Autodesk Inventor part; units mm, degrees
ref_plane "YZ Plane" through (0, 0, 0) normal (1, 0, 0) x (0, 1, 0)
ref_plane "XZ Plane" through (0, 0, 0) normal (0, 1, 0) x (-1, 0, 0)
ref_plane "XY Plane" through (0, 0, 0) normal (0, 0, 1) x (1, 0, 0)
sketch "Sketch1" plane through (0, 0, 0) normal (0, 1, 0) x (-1, 0, 0)
  line L0 (-81, 62) -> (81, 62)
  line L1 (81, 62) -> (81, -62)
  line L2 (81, -62) -> (-81, -62)
  line L3 (-81, -62) -> (-81, 62)
  point P0 (0, 0)
  dimension "d117" = 124
  dimension "d118" = 162
  dimension "d119" = 81
  dimension "d120" = 62
extrude "Extrusion1" add sketch "Sketch1" along normal blind 5
fillet "Fillet1" radius 5 4 edges at (81, 2.5, 62) (81, 2.5, -62) (-81, 2.5, -62) (-81, 2.5, 62)
sketch "Sketch3" plane through (0, 5, 0) normal (0, 1, 0) x (1, 0, 0)
  circle A0 centre (74, -55) radius 3
  circle A1 centre (-74, -55) radius 3
  circle A2 centre (-74, 55) radius 3
  circle A3 centre (74, 55) radius 3
  line L0 (-76, -62) -> (76, -62)
  line L1 (81, -57) -> (81, 57)
  line L2 (-81, 57) -> (-81, -57)
  line L3 (76, 62) -> (-76, 62)
  point P0 (0, 0)
  dimension "d121" = 6
  dimension "d122" = 7
  dimension "d123" = 7
  dimension "d124" = 7
  dimension "d125" = 7
hole "Hole1" at (74, 5, 55) at (-74, 5, 55) at (74, 5, -55) at (-74, 5, -55) direction (0, -1, 0) diameter 6 end through all
sketch "Sketch4" plane through (0, 5, 0) normal (0, 1, 0) x (1, 0, 0)
  circle A0 centre (26.1863, -35) radius 5
  circle A1 centre (-26.1863, -35) radius 5
  circle A2 centre (0, 10.5) radius 5
  circle A3 centre (26.1863, 35) radius 5
  circle A4 centre (-26.1863, 35) radius 5
  point P0 (0, 0)
  dimension "d130" = 10
  dimension "d131" = 24.5
  dimension "d132" = 70
  dimension "d133" = 52.3726
  dimension "d134" = 26.1863
  dimension "d135" = 26.1863
  dimension "d136" = 35
hole "Hole2" at (-26.1863, 5, 35) at (26.1863, 5, 35) at (26.1863, 5, -35) at (-26.1863, 5, -35) direction (0, -1, 0) diameter 10 end through all
sketch "Sketch5" plane through (0, 0, 0) normal (0, -1, 0) x (1, 0, 0)
  circle A0 centre (0, 18.5) radius 9
  line L0 (-76, 62) -> (76, 62)
  point P0 (0, 0)
  dimension "d33" = 18
  dimension "d137" = 43.5
extrude "Extrusion3" cut sketch "Sketch5" against normal blind 10
sketch "Sketch7" plane through (0, 5, 0) normal (0, 1, 0) x (1, 0, 0)
  line L0 (9, 37) -> (-9, 37)
  line L1 (-9, 37) -> (-9, 72)
  line L2 (-9, 72) -> (9, 72)
  line L3 (9, 72) -> (9, 37)
  line L4 (76, 62) -> (-76, 62)
  point P0 (0, 0)
  point P1 (9, 62)
  point P2 (-9, 62)
  dimension "d138" = 35
  dimension "d139" = 10
  dimension "d140" = 18
  dimension "d141" = 9
extrude "Extrusion5" cut sketch "Sketch7" against normal through all contours L0 L1 L4 L3
sketch "Sketch9" plane through (0, 5, 0) normal (0, 1, 0) x (1, 0, 0)
  circle A0 centre (-8.5, -49.5) radius 1.5
  circle A1 centre (8.5, -49.5) radius 1.5
  line L0 (-76, -62) -> (76, -62)
  line L1 (81, -57) -> (81, 57)
  line L2 (-81, 57) -> (-81, -57)
  dimension "d51" = 3
  dimension "d53" = 3
  dimension "d142" = 12.5
  dimension "d143" = 72.5
  dimension "d144" = 72.5
hole "Hole4" at (-8.5, 5, 49.5) at (8.5, 5, 49.5) direction (0, -1, 0) diameter 5 end through all
sketch "Sketch10" plane through (0, 5, 0) normal (0, 1, 0) x (1, 0, 0)
  circle A0 centre (0, -40) radius 3
  line L0 (-76, -62) -> (76, -62)
  point P0 (0, 0)
  dimension "d64" = 6
  dimension "d145" = 22
hole "Hole5" at (0, 5, 40) direction (0, -1, 0) diameter 6 depth 20 tip angle 118
sketch "Sketch13" plane through (0, 5, 0) normal (0, 1, 0) x (1, 0, 0)
  circle A0 centre (-66, 18) radius 2
  line L0 (-92, 62) -> (-157, 62) construction
  line L1 (-81, 110) -> (-81, -20) construction
  circle A1 centre (-66, 12) radius 2
  circle A2 centre (-66, 6) radius 2
  circle A3 centre (-66, 0) radius 2
  circle A4 centre (-66, -6) radius 2
  circle A5 centre (-66, -12) radius 2
  circle A6 centre (-66, -18) radius 2
  circle A7 centre (-60, 18) radius 2
  circle A8 centre (-60, 12) radius 2
  circle A9 centre (-60, 6) radius 2
  circle A10 centre (-60, 0) radius 2
  circle A11 centre (-60, -6) radius 2
  circle A12 centre (-60, -12) radius 2
  circle A13 centre (-60, -18) radius 2
  circle A14 centre (-54, 18) radius 2
  circle A15 centre (-54, 12) radius 2
  circle A16 centre (-54, 6) radius 2
  circle A17 centre (-54, 0) radius 2
  circle A18 centre (-54, -6) radius 2
  circle A19 centre (-54, -12) radius 2
  circle A20 centre (-54, -18) radius 2
  circle A21 centre (-48, 18) radius 2
  circle A22 centre (-48, 12) radius 2
  circle A23 centre (-48, 6) radius 2
  circle A24 centre (-48, 0) radius 2
  circle A25 centre (-48, -6) radius 2
  circle A26 centre (-48, -12) radius 2
  circle A27 centre (-48, -18) radius 2
  circle A28 centre (-42, 18) radius 2
  circle A29 centre (-42, 12) radius 2
  circle A30 centre (-42, 6) radius 2
  circle A31 centre (-42, 0) radius 2
  circle A32 centre (-42, -6) radius 2
  circle A33 centre (-42, -12) radius 2
  circle A34 centre (-42, -18) radius 2
  circle A35 centre (-36, 18) radius 2
  circle A36 centre (-36, 12) radius 2
  circle A37 centre (-36, 6) radius 2
  circle A38 centre (-36, 0) radius 2
  circle A39 centre (-36, -6) radius 2
  circle A40 centre (-36, -12) radius 2
  circle A41 centre (-36, -18) radius 2
  circle A42 centre (-30, 18) radius 2
  circle A43 centre (-30, 12) radius 2
  circle A44 centre (-30, 6) radius 2
  circle A45 centre (-30, 0) radius 2
  circle A46 centre (-30, -6) radius 2
  circle A47 centre (-30, -12) radius 2
  circle A48 centre (-30, -18) radius 2
  line L2 (-81, 57) -> (-81, -57)
  line L3 (-9, 62) -> (-76, 62)
  point P0 (0, 0)
  dimension "d101" = 44
  dimension "d102" = 15
  dimension "d103" = 4
  dimension "d106" = 6
  dimension "d109" = 6
  dimension "d146" = 0
  dimension "d147" = 0
extrude "Extrusion7" cut sketch "Sketch13" against normal through all
equation "\"d68\" = d64"
properties part number "x_axis_plate_top_t" material "PET Plastic"
The model under review builds one solid part; all positions refer to its coordinate system, in mm. Give positions to 0.01 mm unless a question says otherwise; leave off trailing zeros. Write each loop counter-clockwise with the first axis right and the second up, starting at its lowest first coordinate (ties: lowest second). Pieces come first, ordered by that corner, then holes. Notation, with made-up numbers: M 64.25,-10 L 96.25,-10 A36 ccw 96.25,26 Z; hole C 41,-37.5 d10. An arc over 180 degrees is marked long. Write each question's results on one line, items separated by ' | '. Start each with the question number.
1. We need section B-B (x = -42). Count the separate pieces of the cut face and the enclosed holes in it, and give its area (3 significant figures).
2. We need section A-A (z = 49.5). Write out the cut boundary in (x, y), and give its area (3 significant figures).
3. For probe 1 along X at (y, z) = (1.9, -47.5); probe 2 along Z at (x, y) = (2, 3.95); probe 3 along Z at (x, y) = (25, 3.15), list the stretches that pass through material, from the lowest coordinate up. Write a range as [from, to].
4. Mouldability with a two-part tool opening along X and no side actions: class faces 1 (the flat face through (-81, 2, 1)), 2 (the cylindrical face through (-58.925, 2.535, 16.314)), 3 (the cylindrical face through (79, 3, 61)) as released by +X, released by -X, zero draft, split by the parting line, or undercut.
5. Insertion check: pin 1 Ø3 at (x, z) = (-36, 0) entering from +Y; pin 2 Ø1.5 at (x, y) = (0, 1.5) entering from -Z. Each pin has a flat end and moves straight along its axis. Give the tip position at first contact, or say it passes through.
6. We need section D-D (z = -35). Write out the cut boundary in (x, y).
Results found:
1) separate pieces: 8 | enclosed holes: 0 | area: 480 mm^2
2) outline: M -81,0 L -11,0 L -11,5 L -81,5 Z; M -6,0 L 6,0 L 6,5 L -6,5 Z; M 11,0 L 81,0 L 81,5 L 11,5 Z | area: 760 mm^2
3) probe 1: x = [-81, -9], [9, 81] | probe 2: z = [-37, 9.73], [27.27, 37.76], [42.24, 62] | probe 3: z = [-62, -39.86], [-30.14, 30.14], [39.86, 62]
4) face 1: released by -X | face 2: undercut | face 3: released by +X
5) pin 1: passes through | pin 2: stops at z = -37
6) outline: M -81,0 L -31.19,0 L -31.19,5 L -81,5 Z; M -21.19,0 L 21.19,0 L 21.19,5 L -21.19,5 Z; M 31.19,0 L 81,0 L 81,5 L 31.19,5 Z
